from build123d import *

# Parameters (mm, degrees)
SKETCH1_W               = 36
SKETCH1_H               = 9
BOSS_EXTRUDE1_DEPTH     = 28
CUT_EXTRUDE1_DEPTH      = 28
CUT_EXTRUDE2_DEPTH      = 36
SKETCH5_W               = 11.440376565
SKETCH5_H               = 15.618965423
CUT_EXTRUDE4_DEPTH      = 2
CUT_EXTRUDE5_DEPTH      = 2
CUT_EXTRUDE5_DEPTH_BACK = 2
CUT_EXTRUDE6_DEPTH      = 26
CUT_EXTRUDE7_DEPTH      = 26
SKETCH10_R              = 3
CUT_EXTRUDE8_DEPTH      = 7
SKETCH11_R              = 1.5
CUT_EXTRUDE9_DEPTH      = 2
SKETCH12_R              = 1.5
CUT_EXTRUDE10_DEPTH     = 9
SKETCH13_R              = 3
CUT_EXTRUDE11_DEPTH     = 7


with BuildPart() as part:
    # Sketch1 → Boss-Extrude1 (new body)
    with BuildSketch(Plane.XY):
        with Locations((18, 4.5)):
            Rectangle(SKETCH1_W, SKETCH1_H)
    extrude(amount=BOSS_EXTRUDE1_DEPTH)

    # Sketch2 → Cut-Extrude1 (cut)
    with BuildSketch(Plane.XY):
        Polygon((0, 4.5), (4.5, 9), (0, 9), align=None)
        Polygon((36, 4.5), (31.5, 9), (36, 9), align=None)
    extrude(amount=CUT_EXTRUDE1_DEPTH, mode=Mode.SUBTRACT)

    # Sketch3 → Cut-Extrude2 (cut)
    with BuildSketch(Plane(origin=(0, 0, 0), x_dir=(0, 0, -1), z_dir=(1, 0, 0))):
        Polygon((-28, 4.5), (-23.5, 9), (-28, 9), align=None)
    extrude(amount=CUT_EXTRUDE2_DEPTH, mode=Mode.SUBTRACT)

    # Sketch5 → Cut-Extrude4 (cut)
    with BuildSketch(Plane(origin=(32, 0, 32), x_dir=(0, 1, 0), z_dir=(0.707106781, 0, 0.707106781))):
        with Locations((5.720188283, -5.935696583)):
            Rectangle(SKETCH5_W, SKETCH5_H)
    extrude(amount=-CUT_EXTRUDE4_DEPTH, mode=Mode.SUBTRACT)

    # Sketch6 → Cut-Extrude5 (cut, two sides)
    with BuildSketch(Plane(origin=(4, 0, -4), x_dir=(0.577350269, -0.577350269, 0.577350269), z_dir=(-0.707106781, 0, 0.707106781))) as cut_extrude5_sk:
        Polygon((26.558112383, 29.802125204), (32.719347855, 28.647424665), (30.19862658, 32.212262879), align=None)
    extrude(amount=CUT_EXTRUDE5_DEPTH, mode=Mode.SUBTRACT)
    extrude(cut_extrude5_sk.sketch, amount=-CUT_EXTRUDE5_DEPTH_BACK, mode=Mode.SUBTRACT)

    # Sketch7 → Cut-Extrude6 (cut)
    with BuildSketch(Plane.XY):
        Polygon((5, 0), (5, 3), (5.707106781, 3.707106781), (13.104524105, 3.707106781), (13.811630886, 3), (13.811630886, 0), align=None)
    extrude(amount=CUT_EXTRUDE6_DEPTH, mode=Mode.SUBTRACT)

    # Sketch8 → Cut-Extrude7 (cut)
    with BuildSketch(Plane.XY.offset(28)):
        Polygon((36, 0), (30, 0), (34.5, 4.5), (34.5, 6), (36, 6), align=None)
    extrude(amount=-CUT_EXTRUDE7_DEPTH, mode=Mode.SUBTRACT)

    # Sketch10 → Cut-Extrude8 (cut)
    with BuildSketch(Plane(origin=(0, 9, 0), x_dir=(1, 0, 0), z_dir=(0, 1, 0))):
        with Locations((22, -6.5)):
            Circle(SKETCH10_R)
    extrude(amount=-CUT_EXTRUDE8_DEPTH, mode=Mode.SUBTRACT)

    # Sketch11 → Cut-Extrude9 (cut)
    with BuildSketch(Plane(origin=(0, 2, 0), x_dir=(1, 0, 0), z_dir=(0, 1, 0))):
        with Locations((22, -6.5)):
            Circle(SKETCH11_R)
    extrude(amount=-CUT_EXTRUDE9_DEPTH, mode=Mode.SUBTRACT)

    # Sketch12 → Cut-Extrude10 (cut)
    with BuildSketch(Plane(origin=(0, 0, 0), x_dir=(1, 0, 0), z_dir=(0, 1, 0))):
        with Locations((22, -16.5)):
            Circle(SKETCH12_R)
    extrude(amount=CUT_EXTRUDE10_DEPTH, mode=Mode.SUBTRACT)

    # Sketch13 → Cut-Extrude11 (cut)
    with BuildSketch(Plane(origin=(0, 9, 0), x_dir=(1, 0, 0), z_dir=(0, 1, 0))):
        with Locations((22, -16.5)):
            Circle(SKETCH13_R)
    extrude(amount=-CUT_EXTRUDE11_DEPTH, mode=Mode.SUBTRACT)


solid = part.part
Could you check a few things on this model? Use its own coordinates, in mm. A direction names the side the tool comes from. Coordinates: 2 decimals unless noted, no trailing zeros. Write each loop counter-clockwise with the first axis right and the second up, starting at its lowest first coordinate (ties: lowest second). Pieces come first, ordered by that corner, then holes. Notation, with made-up numbers: (25, -32) - (60, -32) arc R12 ccw to (60, -22) - close; hole circle Ø3 at (14, 57.25). An arc over 180 degrees is marked (long way). Write item = value, one per line.
1) Will these pins go through, and if not, where does the flat tip stop? pin 1 Ø3.5 at (x, z) = (22, 16.5) entering from +Y; pin 2 Ø1.5 at (y, z) = (2, 12) entering from +X; pin 3 Ø3 at (x, y) = (8, 2) entering from -Z; pin 4 Ø1.8 at (x, z) = (22, 6.5) entering from +Y.
Result set:
pin_1 = 2
pin_2 = 32.75
pin_3 = 26
pin_4 = through
2) For faces 5 (the cylindrical face through (19.79, 5.55, 4.47)), 6 (the flat face through (36, 2, 1)), 7 (the flat face through (13.812, 2, 13)), 8 (the flat face through (16, 2, 28)), 9 (the flat face through (34, 2, 2)), which set-ups out of +Z, -Z, +X, -X, +Y, -Y let a thin tool reach every point of the face, with its end or its side?
Result set:
face_5 = +Y
face_6 = +Z, -Z, +X, +Y, -Y
face_7 = -Z, -Y
face_8 = +Z, +X, -X, +Y, -Y
face_9 = +Z, +X, -Y
3) Please list where these lines run through material, in increasing order: line 1 (Z direction, x = 22, y = 1.65); line 2 (Z direction, x = 22, y = 5.5); line 3 (X direction, y = 3.5, z = 17.75). Write a range as [from, to].
Result set:
line_1 = [0, 5], [8, 15], [18, 28]
line_2 = [0, 3.5], [9.5, 13.5], [19.5, 27]
line_3 = [0, 5.5], [13.31, 19.27], [24.73, 33.5]
4) Suppose I cut it at A-A on x = 22. Please give me the cut outline in (y, z).
Result set:
outline = (0, 0) - (9, 0) - (9, 3.5) - (2, 3.5) - (2, 5) - (0, 5) - close; (0, 8) - (2, 8) - (2, 9.5) - (9, 9.5) - (9, 13.5) - (2, 13.5) - (2, 15) - (0, 15) - close; (0, 18) - (2, 18) - (2, 19.5) - (9, 19.5) - (9, 23.5) - (4.5, 28) - (0, 28) - close
5) Suppose I cut it at D-D on z = 12.5. Please give me the cut outline in (x, y).
Result set:
outline = (0, 0) - (5, 0) - (5, 3) - (5.71, 3.71) - (13.1, 3.71) - (13.81, 3) - (13.81, 0) - (30, 0) - (34.5, 4.5) - (34.5, 6) - (31.5, 9) - (4.5, 9) - (0, 4.5) - close
6) Suppose I cut it at C-C on y = 8.5. Please give me the cut outline in (x, z), plus the area to 3 significant figures.
Result set:
outline = (4, 0) - (32, 0) - (32, 23.69) - (31.69, 24) - (4, 24) - close; hole circle Ø6 at (22, 6.5); hole circle Ø6 at (22, 16.5)
area = 615 mm2
7) We'd pull the mould along X, two halves only. Please class faces 1 (the flat face through (18, 0, 14)), 2 (the flat face through (9, 2, 26)), 3 (the flat face through (2.2, 6.7, 13.8)), 4 (the flat face through (34.5, 5, 15)): +X half, -X half, draft (parallel to the pull), parting line (faces both ways), or undercut.
Result set:
face_1 = draft
face_2 = undercut
face_3 = -X half
face_4 = +X half
8) Suppose I cut it at B-B on z = 16.5. Please give me the cut outline in (x, y), plus the area to 3 significant figures.
Result set:
outline = (0, 0) - (5, 0) - (5, 3) - (5.71, 3.71) - (13.1, 3.71) - (13.81, 3) - (13.81, 0) - (20.5, 0) - (20.5, 2) - (19, 2) - (19, 9) - (4.5, 9) - (0, 4.5) - close; (23.5, 0) - (30, 0) - (34.5, 4.5) - (34.5, 6) - (31.5, 9) - (25, 9) - (25, 2) - (23.5, 2) - close
area = 206 mm2
